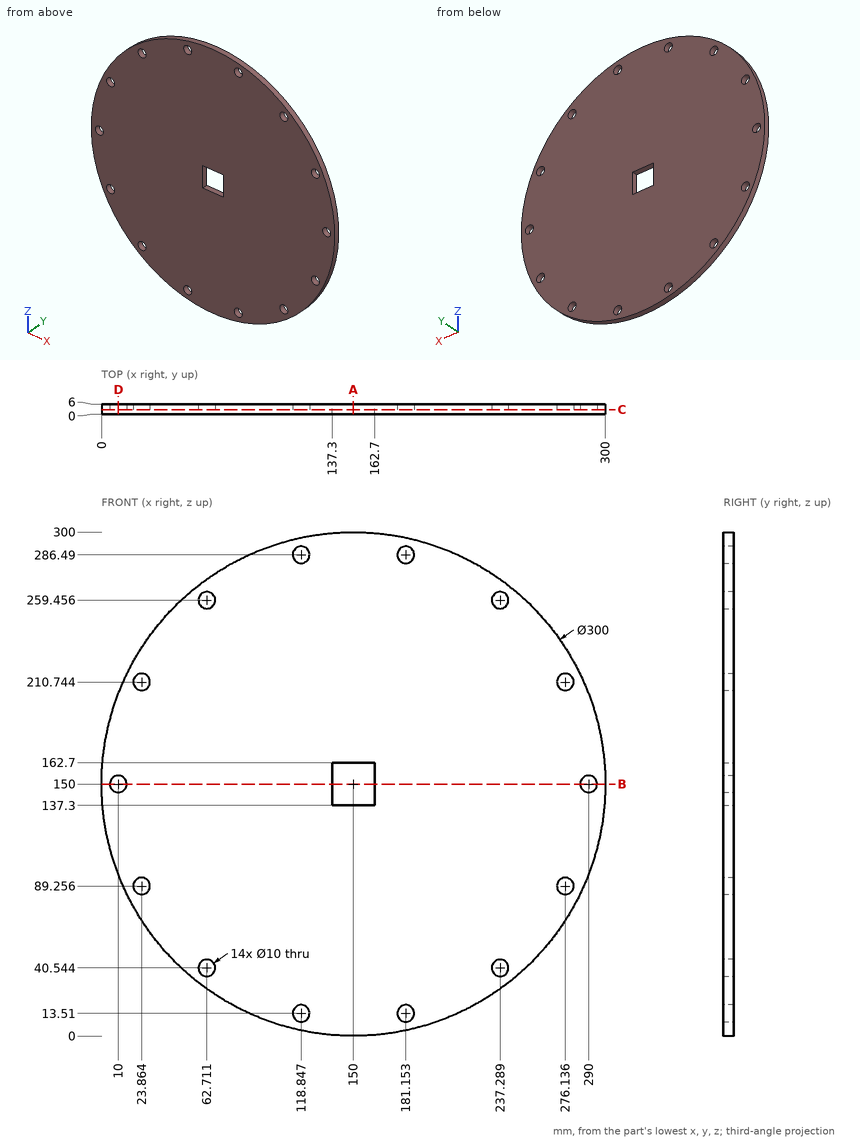
Answer from the drawing. Dimensions are ordinates in mm from the lowest x, y and z of the part. Coordinates: 2 decimals unless noted, no trailing zeros. Write each loop counter-clockwise with the first axis right and the second up, starting at its lowest first coordinate (ties: lowest second). Pieces come first, ordered by that corner, then holes. Notation, with made-up numbers: M -36,-11 L -15,-11 A17 cw -15,21 Z; hole C 15,-9 d1. An arc over 180 degrees is marked long. Put each result on its own line as item: value. Start each with the question number.
1. A cutting plane is placed at D-D on x = 10. Write down the section's boundary in (y, z).
2. Consider line 1 (X direction, y = 1.45, z = 150); line 2 (Z direction, x = 149, y = 3.9); line 3 (X direction, y = 4.1, z = 86). Determine where each line is inside the solid, lowest interval first. Write a range as from..to.
3. A cutting plane is placed at A-A on x = 150. Write down the section's boundary in (y, z).
4. Flat-ended cylindrical pins translate along their axes: P1, Ø4, axis at x = 136.5, z = 48, coming from the -Y side; P2, Ø3, axis at y = 3.5, z = 154.5, coming from the +X side; P3, Ø1, axis at y = 5, z = 229, coming from the -X side. Find the tip coordinate at first contact, or state that the pin passes through.
5. A cutting plane is placed at C-C on y = 2.6. Count the separate pieces of the cut face and the enclosed holes in it, then the cut area to 3 significant figures.
6. A cutting plane is placed at B-B on z = 150. Write down the section's boundary in (x, y).
Resolved:
1. outline: M 0,96.15 L 6,96.15 L 6,145 L 0,145 Z; M 0,155 L 6,155 L 6,203.85 L 0,203.85 Z
2. line 1: x = 0..5, 15..137.3, 162.7..285, 295..300
2. line 2: z = 0..137.3, 162.7..300
2. line 3: x = 14.34..20.07, 27.66..272.34, 279.93..285.66
3. outline: M 0,0 L 6,0 L 6,137.3 L 0,137.3 Z; M 0,162.7 L 6,162.7 L 6,300 L 0,300 Z
4. P1: stops at y = 0
4. P2: stops at x = 299.97
4. P3: stops at x = 22.18
5. separate pieces: 1
5. enclosed holes: 15
5. area: 68,900 mm2
6. outline: M 0,0 L 5,0 L 5,6 L 0,6 Z; M 15,0 L 137.3,0 L 137.3,6 L 15,6 Z; M 162.7,0 L 285,0 L 285,6 L 162.7,6 Z; M 295,0 L 300,0 L 300,6 L 295,6 Z
